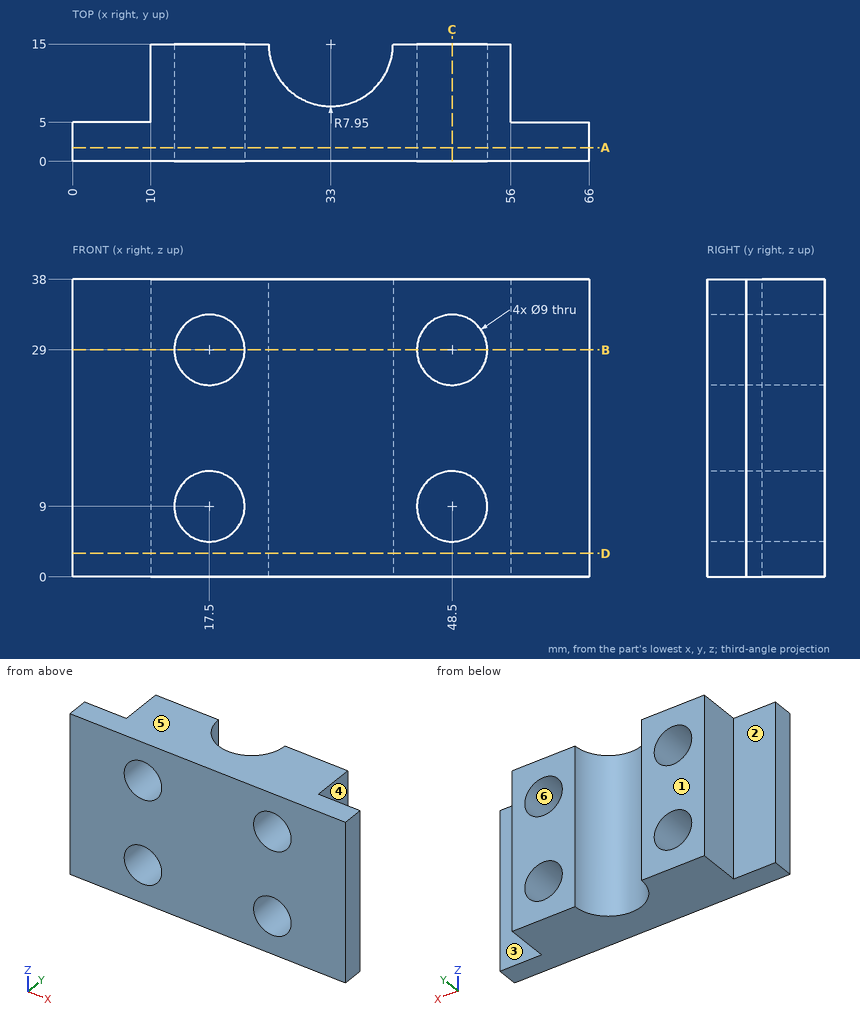
Design review of the part shown in the three views and the two pictorial views. Dimensions are in mm from the part's minimum x, y and z. A direction names the side the tool comes from. Give positions to 0.01 mm unless a question says otherwise; leave off trailing zeros. Write each loop counter-clockwise with the first axis right and the second up, starting at its lowest first coordinate (ties: lowest second). Pieces come first, ordered by that corner, then holes. Notation, with made-up numbers: (41, 13) -> (63, 13) arc R31 cw to (63, 42) -> close; hole circle Ø11 at (47, 69.5). An arc over 180 degrees is marked (long way). Answer in a Markdown table with one row per item.
1) Add section A-A on y = 1.75. State the section outline as (x, z) points, plus the area to 3 significant figures.
Worked answers:
| item | result |
|---|---|
| outline | (0, 0) -> (66, 0) -> (66, 38) -> (0, 38) -> close; hole circle Ø9 at (17.5, 9); hole circle Ø9 at (17.5, 29); hole circle Ø9 at (48.5, 9); hole circle Ø9 at (48.5, 29) |
| area | 2,250 mm² |
2) Clearance check with flat-ended pins moving along their axes: P1, Ø3, axis at y = 10, z = 23.5, coming from the -X side; P2, Ø3, axis at x = 59.5, z = 21, coming from the +Y side; P3, Ø1, axis at x = 28.5, z = 21, coming from the +Y side. State where each tip first meets the part, or that it passes through.
Worked answers:
| item | result |
|---|---|
| P1 | x = 10 |
| P2 | y = 5 |
| P3 | y = 8.82 |
3) Tool access review of the marked faces 1, 2 and 3: name each direction out of +Z, -Z, +X, -X, +Y, -Y from which nothing blocks a thin tool from reaching the whole face with its end or side.
Worked answers:
| item | result |
|---|---|
| face 1 | +Z, -Z, +X, -X, +Y |
| face 2 | +Z, -Z, -X, +Y |
| face 3 | +Z, -Z, +X, +Y |
4) Add section B-B on z = 29. State the section outline as (x, y) points, plus the area to 3 significant figures.
Worked answers:
| item | result |
|---|---|
| outline | (0, 0) -> (13, 0) -> (13, 15) -> (10, 15) -> (10, 5) -> (0, 5) -> close; (22, 0) -> (44, 0) -> (44, 15) -> (40.95, 15) arc R7.95 cw to (25.05, 15) -> (22, 15) -> close; (53, 0) -> (66, 0) -> (66, 5) -> (56, 5) -> (56, 15) -> (53, 15) -> close |
| area | 421 mm² |
5) Mouldability with a two-part tool opening along Z and no side actions: class the marked faces 4, 5 and 6 as +Z half, -Z half, draft (parallel to the pull), parting line (faces both ways), or undercut.
Worked answers:
| item | result |
|---|---|
| face 4 | draft |
| face 5 | +Z half |
| face 6 | undercut |
6) Add section C-C on x = 48.5. State the section outline as (y, z) points.
Worked answers:
| item | result |
|---|---|
| outline | (0, 0) -> (15, 0) -> (15, 4.5) -> (0, 4.5) -> close; (0, 13.5) -> (15, 13.5) -> (15, 24.5) -> (0, 24.5) -> close; (0, 33.5) -> (15, 33.5) -> (15, 38) -> (0, 38) -> close |
7) For L1, parallel to X at y = 3.5, z = 9; L2, parallel to Z at x = 48.5, y = 4.75; L3, parallel to X at y = 14.5, z = 19, list the stretches that pass through material, from the lowest coordinate up. Write a range as [from, to].
Worked answers:
| item | result |
|---|---|
| L1 | [0, 13], [22, 44], [53, 66] |
| L2 | [0, 4.5], [13.5, 24.5], [33.5, 38] |
| L3 | [10, 25.07], [40.93, 56] |
8) Add section D-D on z = 3. State the section outline as (x, y) points, plus the area to 3 significant figures.
Worked answers:
| item | result |
|---|---|
| outline | (0, 0) -> (66, 0) -> (66, 5) -> (56, 5) -> (56, 15) -> (40.95, 15) arc R7.95 cw to (25.05, 15) -> (10, 15) -> (10, 5) -> (0, 5) -> close |
| area | 691 mm² |
